Check sheet for the modelled part. Datum: model origin and axes. Units: mm. Round coordinates to 2 decimals unless told otherwise and drop trailing zeros. Write each loop counter-clockwise with the first axis right and the second up, starting at its lowest first coordinate (ties: lowest second). Pieces come first, ordered by that corner, then holes.
Item 1: Depth check by flat-ended pin: pin 1 (5 mm diameter, centred on x = 29, z = -15.5, fed in from +Y); pin 2 (2.5 mm diameter, centred on x = 8, z = 8, fed in from +Y). Enter the tip coordinate at first touch or a pass-through.
Item 2: Section check B-B, the plane x = -24.5. Record the cut outline in (y, z).
Item 3: Section check A-A, the plane x = 39. Record the cut outline in (y, z), plus the area to 3 significant figures.
Item 4: Release check for a two-part mould opening along Z. For faces 1 (the cylindrical face through (-42.14, 1.51, -21.6)), 2 (the conical face through (5.7, 0.17, 10.6)), 3 (the cylindrical face through (38.521, 1.479, 19.655)), 4 (the conical face through (-41.675, 2.604, 21.213)) record: pulls with the +Z half, pulls with the -Z half, needs draft (parallel to the pull), parting line crosses it, or undercut.
Item 5: Material ranges on line 1 along Z through (x, y) = (31, 1.6); line 2 along Z through (x, y) = (-31, 1.5); line 3 along X through (y, z) = (3.65, 8), recorded low to high.
Item 6: Section check C-C, the plane z = 18.5. State how many separate pieces and enclosed holes the cut face has, plus the area to 3 significant figures.
from build123d import *
from build123d.topology import SkipClean

# Parameters (mm, degrees)
SKETCH1_W           = 86
SKETCH1_H           = 45
SKETCH1_R           = 1.25
BOSS_EXTRUDE1_DEPTH = 3
FILLET1_R           = 3
SKETCH2_R           = 1.5
CUT_EXTRUDE1_DEPTH  = 49.623553963
SHELL1_T            = -2.8
RIB1_REACH          = 50.624
CUT_EXTRUDE2_DEPTH  = 49.623553963
BOSS_EXTRUDE2_START = 1
SKETCH5_R           = 4.3
SKETCH5_R_2         = 1.5
BOSS_EXTRUDE2_DEPTH = 1
CHAMFER1_SIZE       = 1


with BuildPart() as part:
    # Sketch1 → Boss-Extrude1 (new body)
    with BuildSketch(Plane(origin=(0, 0, 0), x_dir=(1, 0, 0), z_dir=(0, 1, 0))):
        Rectangle(SKETCH1_W, SKETCH1_H)
        with Locations(Location((-39, 18.5, 0), (0, 0, 270))):
            Circle(SKETCH1_R, mode=Mode.SUBTRACT)
        with Locations(Location((39, 18.5, 0), (0, 0, 270))):
            Circle(SKETCH1_R, mode=Mode.SUBTRACT)
        with Locations(Location((39, -18.5, 0), (0, 0, 270))):
            Circle(SKETCH1_R, mode=Mode.SUBTRACT)
        with Locations(Location((-39, -18.5, 0), (0, 0, 270))):
            Circle(SKETCH1_R, mode=Mode.SUBTRACT)
    extrude(amount=BOSS_EXTRUDE1_DEPTH)

    # Fillet1
    fillet1_edges = [part.edges().sort_by_distance(p)[0] for p in [
        (43, 1.5, 22.5),
        (-43, 1.5, 22.5),
        (-43, 1.5, -22.5),
        (43, 1.5, -22.5),
    ]]
    fillet(fillet1_edges, radius=FILLET1_R)

    # Sketch2 → Cut-Extrude1 (cut, through all)
    with BuildSketch(Plane(origin=(0, 3, 0), x_dir=(1, 0, 0), z_dir=(0, 1, 0))):
        with Locations(Location((8, -8, 0), (0, 0, 270))):
            Circle(SKETCH2_R)
        with Locations(Location((-8, -8, 0), (0, 0, 270))):
            Circle(SKETCH2_R)
    extrude(amount=-CUT_EXTRUDE1_DEPTH, mode=Mode.SUBTRACT)

    # Shell1
    shell1_openings = [part.faces().sort_by_distance(p)[0] for p in [
        (0, 3, -0.029540883),
    ]]
    offset(amount=SHELL1_T, openings=shell1_openings)

    # Sketch3 walls → Rib1 (add, up to next)
    with BuildSketch(Plane(origin=(0, 3, 0), x_dir=(1, 0, 0), z_dir=(0, 1, 0)), mode=Mode.PRIVATE) as rib1_sk1:
        Polygon((-77.783977456, 23.369087639), (9.570170192, -51.304619221), (11.519513639, -49.024255188), (-75.834634008, 25.649451672), align=None)
    rib1_tool1 = extrude(rib1_sk1.sketch, amount=-RIB1_REACH, mode=Mode.PRIVATE) - part.part
    # Sketch3 walls → Rib1 (add, up to next)
    with BuildSketch(Plane(origin=(0, 3, 0), x_dir=(1, 0, 0), z_dir=(0, 1, 0)), mode=Mode.PRIVATE) as rib1_sk2:
        Polygon((-75.930079406, 34.940098058), (22.974178135, -49.60708984), (24.923521582, -47.326725807), (-73.980735959, 37.220462091), align=None)
    rib1_tool2 = extrude(rib1_sk2.sketch, amount=-RIB1_REACH, mode=Mode.PRIVATE) - part.part
    # Sketch3 walls → Rib1 (add, up to next)
    with BuildSketch(Plane(origin=(0, 3, 0), x_dir=(1, 0, 0), z_dir=(0, 1, 0)), mode=Mode.PRIVATE) as rib1_sk3:
        Polygon((26.191376207, -35.254742784), (-71.50019667, 48.255795321), (-73.449540118, 45.975431288), (24.24203276, -37.535106817), align=None)
    rib1_tool3 = extrude(rib1_sk3.sketch, amount=-RIB1_REACH, mode=Mode.PRIVATE) - part.part
    # Sketch3 walls → Rib1 (add, up to next)
    with BuildSketch(Plane(origin=(0, 3, 0), x_dir=(1, 0, 0), z_dir=(0, 1, 0)), mode=Mode.PRIVATE) as rib1_sk4:
        Polygon((41.943939257, -35.56484922), (-56.370030956, 48.47773822), (-58.319374403, 46.197374186), (39.994595809, -37.845213253), align=None)
    rib1_tool4 = extrude(rib1_sk4.sketch, amount=-RIB1_REACH, mode=Mode.PRIVATE) - part.part
    # Sketch3 walls → Rib1 (add, up to next)
    with BuildSketch(Plane(origin=(0, 3, 0), x_dir=(1, 0, 0), z_dir=(0, 1, 0)), mode=Mode.PRIVATE) as rib1_sk5:
        Polygon((-42.364199116, 19.402478496), (40.17566685, -51.155794023), (42.125010297, -48.87542999), (-40.414855668, 21.682842529), align=None)
    rib1_tool5 = extrude(rib1_sk5.sketch, amount=-RIB1_REACH, mode=Mode.PRIVATE) - part.part
    # Sketch3 walls → Rib1 (add, up to next)
    with BuildSketch(Plane(origin=(0, 3, 0), x_dir=(1, 0, 0), z_dir=(0, 1, 0)), mode=Mode.PRIVATE) as rib1_sk6:
        Polygon((-27.344787823, 19.719098562), (56.5220764, -51.973543436), (58.471419848, -49.693179403), (-25.395444376, 21.999462595), align=None)
    rib1_tool6 = extrude(rib1_sk6.sketch, amount=-RIB1_REACH, mode=Mode.PRIVATE) - part.part
    # Sketch3 walls → Rib1 (add, up to next)
    with BuildSketch(Plane(origin=(0, 3, 0), x_dir=(1, 0, 0), z_dir=(0, 1, 0)), mode=Mode.PRIVATE) as rib1_sk7:
        Polygon((-44.38155309, 47.438579234), (68.87285442, -49.375672346), (70.822197867, -47.095308313), (-42.432209642, 49.718943267), align=None)
    rib1_tool7 = extrude(rib1_sk7.sketch, amount=-RIB1_REACH, mode=Mode.PRIVATE) - part.part
    # Sketch3 walls → Rib1 (add, up to next)
    with BuildSketch(Plane(origin=(0, 3, 0), x_dir=(1, 0, 0), z_dir=(0, 1, 0)), mode=Mode.PRIVATE) as rib1_sk8:
        Polygon((-28.60953629, 47.11184298), (71.48616066, -38.453833446), (73.435504108, -36.173469413), (-26.660192843, 49.392207013), align=None)
    rib1_tool8 = extrude(rib1_sk8.sketch, amount=-RIB1_REACH, mode=Mode.PRIVATE) - part.part
    # Sketch3 walls → Rib1 (add, up to next)
    with BuildSketch(Plane(origin=(0, 3, 0), x_dir=(1, 0, 0), z_dir=(0, 1, 0)), mode=Mode.PRIVATE) as rib1_sk9:
        Polygon((-14.02835821, 47.803081759), (73.331762126, -26.875730786), (75.281105573, -24.595366753), (-12.079014763, 50.083445792), align=None)
    rib1_tool9 = extrude(rib1_sk9.sketch, amount=-RIB1_REACH, mode=Mode.PRIVATE) - part.part
    add(rib1_tool1.solids().sort_by_distance((-33.132231908, 3, 12.827583774))[0])
    add(rib1_tool2.solids().sort_by_distance((-25.503278912, 3, 6.193313875))[0])
    add(rib1_tool3.solids().sort_by_distance((-23.629081955, 3, -5.360344252))[0])
    add(rib1_tool4.solids().sort_by_distance((-8.187717573, 3, -5.316262483))[0])
    add(rib1_tool5.solids().sort_by_distance((-0.119594409, 3, 14.736475747))[0])
    add(rib1_tool6.solids().sort_by_distance((15.563316012, 3, 14.987040421))[0])
    add(rib1_tool7.solids().sort_by_distance((13.220322389, 3, -0.17163546))[0])
    add(rib1_tool8.solids().sort_by_distance((22.412983909, 3, -5.469186783))[0])
    add(rib1_tool9.solids().sort_by_distance((30.626373682, 3, -11.603857503))[0])

    # Sketch4 → Cut-Extrude2 (cut, through all)
    with SkipClean():  # the faces are left unmerged after this step: merging them gives an invalid solid
        with BuildSketch(Plane(origin=(0, 3, 0), x_dir=(1, 0, 0), z_dir=(0, 1, 0))):
            with BuildLine():
                Line((-27.401271161, -19.7), (-40.2, -8.759151154))
                Line((-40.2, -8.759151154), (-40.2, -14.631860913))
                ThreePointArc((-40.2, -14.631860913), (-36.136217536, -15.636217536), (-35.131860913, -19.7))
                Line((-35.131860913, -19.7), (-27.401271161, -19.7))
            make_face()
            Polygon((-12.011474131, -19.7), (-40.2, 4.396643081), (-40.2, -4.812412883), (-22.784332052, -19.7), align=None)
            with BuildLine():
                Line((3.378322898, -19.7), (-5.911467584, -11.758727491))
                ThreePointArc((-5.911467584, -11.758727491), (-10.794058942, -11.268521781), (-12.037875863, -6.521636542))
                Line((-12.037875863, -6.521636542), (-37.115109774, 14.915353736))
                ThreePointArc((-37.115109774, 14.915353736), (-38.629377954, 14.466993764), (-40.2, 14.631860913))
                Line((-40.2, 14.631860913), (-40.2, 8.343381352))
                Line((-40.2, 8.343381352), (-7.394535022, -19.7))
                Line((-7.394535022, -19.7), (3.378322898, -19.7))
            make_face()
            with BuildLine():
                Line((18.768119928, -19.7), (9.701138512, -11.949193305))
                ThreePointArc((9.701138512, -11.949193305), (5.205941058, -11.268521781), (3.834243685, -6.933944502))
                Line((3.834243685, -6.933944502), (-27.32244611, 19.7))
                Line((-27.32244611, 19.7), (-35.131860913, 19.7))
                ThreePointArc((-35.131860913, 19.7), (-34.950371139, 18.445172177), (-35.165766327, 17.195717769))
                Line((-35.165766327, 17.195717769), (-10.088532416, -4.241272509))
                ThreePointArc((-10.088532416, -4.241272509), (-5.205941058, -4.731478219), (-3.962124137, -9.478363458))
                Line((-3.962124137, -9.478363458), (7.995262007, -19.7))
                Line((7.995262007, -19.7), (18.768119928, -19.7))
            make_face()
            with BuildLine():
                Line((34.157916958, -19.7), (-11.93264908, 19.7))
                Line((-11.93264908, 19.7), (-22.705507001, 19.7))
                Line((-22.705507001, 19.7), (5.557974977, -4.460718465))
                ThreePointArc((5.557974977, -4.460718465), (10.794058942, -4.731478219), (11.876094115, -9.861691277))
                Line((11.876094115, -9.861691277), (23.385059037, -19.7))
                Line((23.385059037, -19.7), (34.157916958, -19.7))
            make_face()
            with BuildLine():
                Line((40.2, -11.709212236), (3.45714795, 19.7))
                Line((3.45714795, 19.7), (-7.315709971, 19.7))
                Line((-7.315709971, 19.7), (35.340744315, -16.764388341))
                ThreePointArc((35.340744315, -16.764388341), (37.372454935, -14.791415761), (40.2, -14.631860913))
                Line((40.2, -14.631860913), (40.2, -11.709212236))
            make_face()
            Polygon((40.2, 1.446581999), (18.84694498, 19.7), (8.074087059, 19.7), (40.2, -7.762473966), align=None)
            with BuildLine():
                Line((35.131860913, 19.7), (23.463884089, 19.7))
                Line((23.463884089, 19.7), (40.2, 5.393320269))
                Line((40.2, 5.393320269), (40.2, 14.631860913))
                ThreePointArc((40.2, 14.631860913), (36.136217536, 15.636217536), (35.131860913, 19.7))
            make_face()
        extrude(amount=-CUT_EXTRUDE2_DEPTH, mode=Mode.SUBTRACT)

    # Sketch5 → Boss-Extrude2 (add)
    # profile 1 of 2: a face of its own
    with SkipClean():  # the faces are left unmerged after this step: merging them gives an invalid solid
        with BuildSketch(Plane(origin=(0, 3, 0), x_dir=(1, 0, 0), z_dir=(0, 1, 0)).offset(BOSS_EXTRUDE2_START)):
            with Locations(Location((-8, -8, 0), (0, 0, 270))):
                Circle(SKETCH5_R)
            with Locations(Location((-8, -8, 0), (0, 0, 270))):
                Circle(SKETCH5_R_2, mode=Mode.SUBTRACT)
        # profile 2 of 2: a face of its own
        with BuildSketch(Plane(origin=(0, 3, 0), x_dir=(1, 0, 0), z_dir=(0, 1, 0)).offset(BOSS_EXTRUDE2_START)):
            with Locations(Location((8, -8, 0), (0, 0, 270))):
                Circle(SKETCH5_R)
            with Locations(Location((8, -8, 0), (0, 0, 270))):
                Circle(SKETCH5_R_2, mode=Mode.SUBTRACT)
        extrude(amount=-BOSS_EXTRUDE2_DEPTH)

    # Chamfer1
    chamfer1_edges = [part.edges().sort_by_distance(p)[0] for p in [
        (-8, 4, 3.7),
        (8, 4, 3.7),
        (-43, 0, 0),
        (-43, 3, 0),
        (43, 0, 0),
        (0, 0, 22.5),
        (0, 0, -22.5),
        (-42.121320344, 0, 21.621320344),
        (42.121320344, 0, 21.621320344),
        (42.121320344, 0, -21.621320344),
        (-42.121320344, 0, -21.621320344),
        (0, 3, -22.5),
        (43, 3, 0),
        (0, 3, 22.5),
        (-42.121320344, 3, 21.621320344),
        (42.121320344, 3, 21.621320344),
        (42.121320344, 3, -21.621320344),
        (-42.121320344, 3, -21.621320344),
        (5.205941058, 0, 11.268521781),
        (-10.794058942, 0, 11.268521781),
    ]]
    chamfer(chamfer1_edges, length=CHAMFER1_SIZE - 0.0001)  # a hair under: the kernel refuses the full size


solid = part.part
Values found:
1. pin 1: stops at y = 3
1. pin 2: passes through
2. outline: (0, -21.5) - (1, -22.5) - (2, -22.5) - (3, -21.5) - (3, -17.29) - (0, -17.29) - close; (0, -8.08) - (3, -8.08) - (3, -4.13) - (0, -4.13) - close; (0, 5.08) - (3, 5.08) - (3, 9.02) - (0, 9.02) - close; (0, 18.23) - (3, 18.23) - (3, 21.5) - (2, 22.5) - (1, 22.5) - (0, 21.5) - close
3. outline: (0, -21.5) - (1, -22.5) - (2, -22.5) - (3, -21.5) - (3, -19.75) - (0, -19.75) - close; (0, -17.25) - (3, -17.25) - (3, -14.45) - (0, -14.45) - close; (0, -6.42) - (3, -6.42) - (3, -2.47) - (0, -2.47) - close; (0, 6.74) - (3, 6.74) - (3, 10.68) - (0, 10.68) - close; (0, 14.45) - (3, 14.45) - (3, 17.25) - (0, 17.25) - close; (0, 19.75) - (3, 19.75) - (3, 21.5) - (2, 22.5) - (1, 22.5) - (0, 21.5) - close
3. area: 55.0 mm2
4. face 1: pulls with the -Z half
4. face 2: undercut
4. face 3: undercut
4. face 4: pulls with the +Z half
5. line 1: z = -22.5 to -19.7, -13.26 to -9.31, -0.1 to 3.84, 13.05 to 17, 19.7 to 22.5
5. line 2: z = -22.5 to -19.7, -13.63 to -9.69, -0.48 to 3.47, 12.68 to 16.62, 19.7 to 22.5
5. line 3: x = -11.65 to -9.5, -6.5 to -4.35, 4.35 to 6.5, 9.5 to 11.65
6. separate pieces: 8
6. enclosed holes: 0
6. area: 93.3 mm2
